The listing builds one solid part. Answer for the finished solid, in the listing's coordinates (mm). Face numbers are marked on the shaded views. A direction names the side the tool comes from. Round coordinates to 2 decimals unless told otherwise and drop trailing zeros. Loops run counter-clockwise (first coordinate to the right, second up) from the corner with the lowest first, then second, coordinate; pieces in that order, holes last. Notation, with made-up numbers: (30.5, 26.5) -> (84.5, 26.5) arc R19 cw to (84.5, 36.5) -> close; hole circle Ø4 at (61, 3.25). An arc over 180 degrees is marked (long way). Use a Markdown table: item, result. Add a question column.
Q1. Section A-A on x = 0 is taken. Give the vertices of the cut face in (y, z), then the cut area to 3 significant figures.
Q2. Given pin 1 Ø1.5 at (y, z) = (-2, 14) entering from -X; pin 2 Ø3 at (y, z) = (-2, 11.5) entering from -X; pin 3 Ø5 at (x, z) = (1, 15) entering from +Y, each flat-ended and moving along its own axis, determine where each tip first touches the part or whether it passes through.
Q3. Section C-C on x = 3 is taken. Give the vertices of the cut face in (y, z).
Q4. Section D-D on y = -7.25 is taken. Give the vertices of the cut face in (x, z).
Q5. Section B-B on z = 6.25 is taken. Give the vertices of the cut face in (x, y), then the cut area to 3 significant figures.
Q6. Which of the six approach directions +Z, -Z, +X, -X, +Y, -Y give full straight-line access (tool end or side, diameter ignored) to the marked faces 5, 6 and 7?
Q7. For a pull along Y with two mould halves and no side action, classify the marked faces 1, 2, 3 and 4 as released by +Y, released by -Y, zero draft, split by the parting line, or undercut.
Q8. Consider line 1 (Y direction, x = -3.5, z = 12.25); line 2 (Y direction, x = 0, z = 4.75); line 3 (Z direction, x = 1.5, y = -3). Determine where each line is inside the solid, lowest interval first.
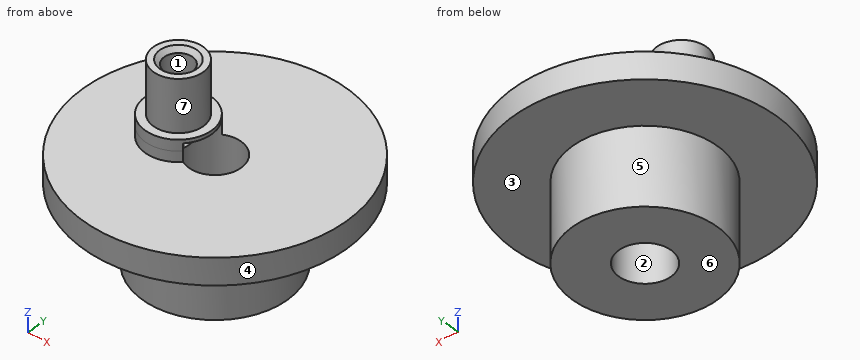
from build123d import *

# Parameters (mm, degrees)
SKETCH1_R                       = 6.9215
SKETCH1_R_2                     = 0.127
BOSS_EXTRUDE1_DEPTH             = 10.922
SKETCH2_R                       = 2.38125
BOSS_EXTRUDE2_DEPTH             = 6.00075
BOSS_EXTRUDE3_START             = -0.762
SKETCH4_R                       = 6.9215
BOSS_EXTRUDE3_DEPTH             = 0.762
SKETCH5_R                       = 3.175
BOSS_EXTRUDE4_DEPTH             = 1.04775
F_6_32_TAPPED_HOLE1_D           = 2.7051
F_6_32_TAPPED_HOLE1_DEPTH       = 7.112
F_6_32_TAPPED_HOLE1_CSINK_D     = 3.556
F_6_32_TAPPED_HOLE1_CSINK_ANGLE = 90
F_6_32_TAPPED_HOLE1_TIP         = 0.81269403
SKETCH9_R                       = 0.127
CUT_EXTRUDE2_DEPTH              = 15.108150995
SKETCH13_R                      = 2.49682
CUT_EXTRUDE5_DEPTH              = 11.6205
SKETCH15_OUTSIDE_W              = 21.02
SKETCH15_OUTSIDE_H              = 21.02
SKETCH15_OUTSIDE_R              = 3.175
CUT_EXTRUDE7_DEPTH              = 1.000000032
BOSS_EXTRUDE6_START             = -2.54
SKETCH16_R                      = 12.573
SKETCH16_R_2                    = 6.9215
BOSS_EXTRUDE6_DEPTH             = 2.54


with BuildPart() as part:
    # Sketch1 → Boss-Extrude1 (new body)
    with BuildSketch(Plane.XY):
        Circle(SKETCH1_R)
        Circle(SKETCH1_R_2, mode=Mode.SUBTRACT)
    extrude(amount=BOSS_EXTRUDE1_DEPTH)

    # Sketch2 → Boss-Extrude2 (add)
    with BuildSketch(Plane.XY.offset(10.922)):
        with Locations((-3.5, 0)):
            Circle(SKETCH2_R)
    extrude(amount=BOSS_EXTRUDE2_DEPTH)

    # Sketch4 → Boss-Extrude3 (add)
    with BuildSketch(Plane.XY.offset(10.922).offset(BOSS_EXTRUDE3_START)):
        Circle(SKETCH4_R)
    extrude(amount=BOSS_EXTRUDE3_DEPTH)

    # Sketch5 → Boss-Extrude4 (add)
    with BuildSketch(Plane.XY.offset(10.922)):
        with Locations(Location((-3.5, 0, 0), (0, 0, 43.593288384))):
            Circle(SKETCH5_R)
    extrude(amount=BOSS_EXTRUDE4_DEPTH)

    # #6-32 Tapped Hole1
    with Locations(Plane.XY.offset(16.92275)):
        with Locations((-3.5, 0)):
            CounterSinkHole(F_6_32_TAPPED_HOLE1_D / 2, F_6_32_TAPPED_HOLE1_CSINK_D / 2, depth=F_6_32_TAPPED_HOLE1_DEPTH, counter_sink_angle=F_6_32_TAPPED_HOLE1_CSINK_ANGLE)
            with Locations((0, 0, -(F_6_32_TAPPED_HOLE1_DEPTH + F_6_32_TAPPED_HOLE1_TIP / 2))):  # 118° drill point
                Cone(0, F_6_32_TAPPED_HOLE1_D / 2, F_6_32_TAPPED_HOLE1_TIP, mode=Mode.SUBTRACT)

    # Sketch9 → Cut-Extrude2 (cut, through all)
    with BuildSketch(Plane(origin=(0, 0, 10.16), x_dir=(-1, 0, 0), z_dir=(0, 0, -1))):
        Circle(SKETCH9_R)
    extrude(amount=-CUT_EXTRUDE2_DEPTH, mode=Mode.SUBTRACT)

    # Sketch13 → Cut-Extrude5 (cut)
    with BuildSketch(Plane(origin=(0, 0, 0), x_dir=(-1, 0, 0), z_dir=(0, 0, -1))):
        Circle(SKETCH13_R)
    extrude(amount=-CUT_EXTRUDE5_DEPTH, mode=Mode.SUBTRACT)

    # Sketch15 outside → Cut-Extrude7 (cut)
    with BuildSketch(Plane.XY.offset(10.922)):
        Rectangle(SKETCH15_OUTSIDE_W, SKETCH15_OUTSIDE_H)
        with Locations(Location((-3.5, 0, 0), (0, 0, 43.593288384))):
            Circle(SKETCH15_OUTSIDE_R, mode=Mode.SUBTRACT)
    extrude(amount=-CUT_EXTRUDE7_DEPTH, mode=Mode.SUBTRACT)

    # Sketch16 → Boss-Extrude6 (add)
    with BuildSketch(Plane.XY.offset(9.921999968).offset(BOSS_EXTRUDE6_START)):
        Circle(SKETCH16_R)
        Circle(SKETCH16_R_2, mode=Mode.SUBTRACT)
    extrude(amount=BOSS_EXTRUDE6_DEPTH)


solid = part.part
Checked values:
| question | item | result |
|---|---|---|
| 1 | outline | (-12.57, 7.38) -> (-6.92, 7.38) -> (-6.92, 0) -> (-2.5, 0) -> (-2.5, 9.92) -> (-12.57, 9.92) -> close; (2.5, 0) -> (6.92, 0) -> (6.92, 7.38) -> (12.57, 7.38) -> (12.57, 9.92) -> (2.5, 9.92) -> close |
| 1 | area | 117 mm2 |
| 2 | pin 1 | stops at x = -5.53 |
| 2 | pin 2 | stops at x = -6.64 |
| 2 | pin 3 | stops at y = 1.29 |
| 3 | outline | (-12.21, 7.38) -> (-6.24, 7.38) -> (-6.24, 0) -> (6.24, 0) -> (6.24, 7.38) -> (12.21, 7.38) -> (12.21, 9.92) -> (-12.21, 9.92) -> close |
| 4 | outline | (-10.27, 7.38) -> (10.27, 7.38) -> (10.27, 9.92) -> (-10.27, 9.92) -> close |
| 5 | outline | circle Ø13.84 at (0, 0); hole circle Ø4.99 at (0, 0) |
| 5 | area | 131 mm2 |
| 6 | face 5 | -Z |
| 6 | face 6 | -Z, +X, -X, +Y, -Y |
| 6 | face 7 | +Z |
| 7 | face 1 | undercut |
| 7 | face 2 | undercut |
| 7 | face 3 | zero draft |
| 7 | face 4 | split by the parting line |
| 8 | line 1 | y = -2.38 to -1.35, 1.35 to 2.38 |
| 8 | line 2 | y = -6.92 to -2.5, 2.5 to 6.92 |
| 8 | line 3 | z = 0 to 9.92 |
